Could you check a few things on this model? Use its own coordinates, in mm. A direction names the side the tool comes from. Give positions to 0.01 mm unless a question says otherwise; leave off trailing zeros. Loops run counter-clockwise (first coordinate to the right, second up) from the corner with the lowest first, then second, coordinate; pieces in that order, holes last. Notation, with made-up numbers: (-11.75, 3) - (-4.75, 3) arc R26 cw to (-4.75, 36) - close; hole circle Ø2 at (-8, 5.5). An arc over 180 degrees is marked (long way). Answer in a Markdown table with one row per item. Add a question column.
Autodesk Inventor part; units mm, degrees
ref_plane "YZ Plane" through (0, 0, 0) normal (1, 0, 0) x (0, 1, 0)
ref_plane "XZ Plane" through (0, 0, 0) normal (0, 1, 0) x (-1, 0, 0)
ref_plane "XY Plane" through (0, 0, 0) normal (0, 0, 1) x (1, 0, 0)
sketch "Sketch1" plane through (0, 0, 0) normal (0, 0, 1) x (1, 0, 0)
  line L0 (0, 0) -> (33.49, 0)
  line L1 (33.49, 0) -> (33.49, 58.49)
  line L2 (33.49, 58.49) -> (0, 58.49)
  line L3 (0, 58.49) -> (0, 0)
  line L4 (-8, 66.49) -> (41.49, 66.49)
  line L5 (41.49, 66.49) -> (41.49, -8)
  line L6 (41.49, -8) -> (-8, -8)
  line L7 (-8, -8) -> (-8, 66.49)
  line L8 (56.49, -8) -> (56.49, 66.49)
  line L9 (41.49, 81.49) -> (-8, 81.49)
  line L10 (-23, 66.49) -> (-23, -8)
  line L11 (-8, -23) -> (41.49, -23)
  circle A0 centre (48.99, 62.49) radius 2.55
  circle A1 centre (48.99, -4) radius 2.55
  circle A2 centre (-15.5, 62.49) radius 2.55
  circle A3 centre (-15.5, -4) radius 2.55
  arc A4 (-8, 81.49) -> (-23, 66.49) centre (-8, 66.49) ccw
  arc A5 (56.49, 66.49) -> (41.49, 81.49) centre (41.49, 66.49) ccw
  arc A6 (41.49, -23) -> (56.49, -8) centre (41.49, -8) ccw
  arc A7 (-23, -8) -> (-8, -23) centre (-8, -8) ccw
  dimension "d0" = 58.49
  dimension "d1" = 33.49
  dimension "d2" = 8
  dimension "d3" = 15
  dimension "d4" = 5.1
  dimension "d5" = 7.5
  dimension "d6" = 5.1
  dimension "d7" = 5.1
  dimension "d8" = 7.5
  dimension "d9" = 5.1
  dimension "d10" = 4
  dimension "d11" = 4
  dimension "d12" = 4
  dimension "d13" = 4
  dimension "d14" = 7.5
  dimension "d15" = 7.5
  dimension "d16" = 15
extrude "Extrusion1" add sketch "Sketch1" against normal blind 46 contours L4 L5 L6 L7
fillet "Fillet1" radius 10 4 edges at (41.49, 66.49, -23) (41.49, -8, -23) (-8, 66.49, -23) (-8, -8, -23)
sketch "Sketch3" plane through (41.49, 2, 0) normal (1, 0, 0) x (0, 0, -1)
  line L0 (46, 56.49) -> (46, -2)
  line L1 (46, 22) -> (42, 22)
  line L2 (42, 22) -> (46, 22)
  line L3 (46, 35) -> (42, 35)
  line L4 (42, 22) -> (42, 35)
  line L5 (0, 54.49) -> (46, 54.49)
  line L6 (46, 65.745) -> (51, 65.745)
  point P0 (0, -2)
  point P1 (44, 22)
  point P2 (44, 35)
  point P3 (48.5, 65.745)
  dimension "d37" = 4
  dimension "d38" = 4
  dimension "d39" = 13
  dimension "d41" = 30.745
extrude "Extrusion3" cut sketch "Sketch3" against normal up to surface (8 mm away)
sketch "Sketch4" plane through (0, 0, -46) normal (0, 0, -1) x (-1, 0, 0)
  line L0 (-86.745, 92.745) -> (53.255, 92.745)
  line L1 (63.255, 82.745) -> (63.255, -24.255)
  line L2 (53.255, -34.255) -> (-86.745, -34.255)
  line L3 (-96.745, -24.255) -> (-96.745, 82.745)
  line L4 (-31.49, -8) -> (-2, -8)
  line L5 (-2, 66.49) -> (-31.49, 66.49)
  line L6 (8, 2) -> (8, 56.49)
  line L7 (-41.49, 56.49) -> (-41.49, 37)
  arc A0 (-86.745, 92.745) -> (-96.745, 82.745) centre (-86.745, 82.745) ccw
  arc A1 (63.255, 82.745) -> (53.255, 92.745) centre (53.255, 82.745) ccw
  arc A2 (53.255, -34.255) -> (63.255, -24.255) centre (53.255, -24.255) ccw
  arc A3 (-96.745, -24.255) -> (-86.745, -34.255) centre (-86.745, -24.255) ccw
  line L8 (53.255, 82.745) -> (-86.745, 82.745)
  line L9 (-86.745, 82.745) -> (-86.745, -24.255)
  line L10 (-86.745, -24.255) -> (53.255, -24.255)
  line L11 (53.255, -24.255) -> (53.255, 82.745)
  circle A4 centre (-86.745, 82.745) radius 2
  circle A5 centre (53.255, 82.745) radius 2
  circle A6 centre (53.255, -24.255) radius 2
  circle A7 centre (-86.745, -24.255) radius 2
  circle A8 centre (-16.745, 82.745) radius 2
  circle A9 centre (-16.745, -24.255) radius 2
  point P0 (0, 0)
  dimension "d46" = 160
  dimension "d47" = 127
  dimension "d48" = 74.49
  dimension "d49" = 49.49
  dimension "d50" = 55.255
  dimension "d51" = 26.255
  dimension "d52" = 10
  dimension "d53" = 10
  dimension "d54" = 107
  dimension "d55" = 140
  dimension "d56" = 4
  dimension "d57" = 4
  dimension "d58" = 4
  dimension "d59" = 4
  dimension "d60" = 4
  dimension "d61" = 4
extrude "Extrusion4" add sketch "Sketch4" along normal blind 3 contours L0 A1 L1 A2 L2 A3 L3 A0 | L8 A8 A5 L11 A6 L10 A9 A7 L9 A4
fillet "Fillet2" radius 8 9 edges at (38.5611, 63.5611, -46) (41.49, 46.745, -46) (-5.0711, 63.5611, -46) (-8, 29.245, -46) (-5.0711, -5.0711, -46) (16.745, -8, -46) (38.5611, -5.0711, -46) (41.49, 13, -46) (16.745, 66.49, -46)
properties part number "Base_Demo_1"
(1) I want a section at A-A on z = -28. Please give me the cut outline in (x, y), then the cut area to 3 significant figures.
(2) We'd pull the mould along Z, two halves only. Please class faces 4 (the cylindrical face through (93.89, 89.74, -47.48)), 5 (the cylindrical face through (16.951, -10.406, -43.719)), 6 (the flat face through (40, 24, -44)): pulls with the +Z half, pulls with the -Z half, needs draft (parallel to the pull), parting line crosses it, or undercut.
(3) On a 3-axis mill with a long thin cutter (end or side, diameter ignored), from which of +Z, -Z, +X, -X, +Y, -Y can I reach the whole of each face in a straight line? I mean faces 1 (the cylindrical face through (-4.99, -5.15, -19.27)), 2 (the cylindrical face through (38.48, 63.64, -19.27)), 3 (the flat face through (0, 30, -23)). Say none if no direction works.
(4) Please list where these lines run through material, in increasing order: line 1 (X direction, y = 27, z = -22); line 2 (Y direction, x = 30.5, z = -6.5); line 3 (Z direction, x = 15, y = -27).
(5) I want a section at D-D on x = -44. Please give me the cut outline in (y, z) (3 decimals).
(6) For pin 1 Ø19 at (y, z) = (25, -18.5) entering from -X; pin 2 Ø2 at (y, z) = (31.5, -33) entering from +X; pin 3 Ø23 at (y, z) = (20, -33) entering from -X, each with a flat end and sliding along its axis, tell me the tip position at first contact or that it passes through.
(7) I want a section at B-B on y = 21.5. Please give me the cut outline in (x, z) (3 decimals), then the cut area to 3 significant figures.
(8) I want a section at C-C on x = 11.5. Please give me the cut outline in (y, z) (3 decimals), then the cut area to 3 significant figures.
Reported:
| question | item | result |
|---|---|---|
| 1 | outline | (-8, 2) arc R10 ccw to (2, -8) - (31.49, -8) arc R10 ccw to (41.49, 2) - (41.49, 56.49) arc R10 ccw to (31.49, 66.49) - (2, 66.49) arc R10 ccw to (-8, 56.49) - close; hole (0, 0) - (33.49, 0) - (33.49, 58.49) - (0, 58.49) - close |
| 1 | area | 1,640 mm² |
| 2 | face 4 | needs draft |
| 2 | face 5 | pulls with the +Z half |
| 2 | face 6 | undercut |
| 3 | face 1 | +Z, -X, -Y |
| 3 | face 2 | +Z, +X, +Y |
| 3 | face 3 | +Z |
| 4 | line 1 | -8 to 0, 33.49 to 41.49 |
| 4 | line 2 | -8 to 0, 58.49 to 66.49 |
| 4 | line 3 | -49 to -46 |
| 5 | outline | (-34.255, -49) - (92.745, -49) - (92.745, -46) - (-34.255, -46) - close |
| 6 | pin 1 | x = -8 |
| 6 | pin 2 | x = 41.49 |
| 6 | pin 3 | x = -11.34 |
| 7 | outline | (-63.255, -49) - (96.745, -49) - (96.745, -46) - (49.49, -46) arc R8 cw to (41.49, -38) - (41.49, 0) - (33.49, 0) - (33.49, -46) - (0, -46) - (0, 0) - (-8, 0) - (-8, -38) arc R8 cw to (-16, -46) - (-63.255, -46) - close |
| 7 | area | 1,240 mm² |
| 8 | outline | (-34.255, -49) - (92.745, -49) - (92.745, -46) - (74.49, -46) arc R8 cw to (66.49, -38) - (66.49, 0) - (58.49, 0) - (58.49, -46) - (0, -46) - (0, 0) - (-8, 0) - (-8, -38) arc R8 cw to (-16, -46) - (-34.255, -46) - close |
| 8 | area | 1,140 mm² |
